Here's how the part is built. I have some questions about the finished solid (model axes, mm). A direction names the side the tool comes from. Coordinates: 2 decimals unless noted, no trailing zeros. Loops run counter-clockwise (first coordinate to the right, second up) from the corner with the lowest first, then second, coordinate; pieces in that order, holes last. Notation, with made-up numbers: M 24.5,51 L 47.5,51 A12 cw 47.5,58 Z; hole C -22,76.25 d1. An arc over 180 degrees is marked long. Use CSV: the item, a comma, the result in double quotes. Start each with the question number.
Q1. If we section it at A-A (z = -52): Please give me the cut outline in (x, y) (3 decimals), and give its area (3 significant figures).
Q2. For pin 1 Ø5 at (y, z) = (6, -34.5) entering from +X; pin 2 Ø1 at (x, y) = (971, 20) entering from -Z, each with a flat end and sliding along its axis, tell me the tip position at first contact or that it passes through.
Q3. If we mould it in two halves opening along Z, with no side actions, what happens to faces 1 (the flat face through (604, 22.225, -38)), 2 (the flat face through (37.9, 2.4, -38.3)), 3 (the flat face through (604, 25.4, -38))? For each: +Z half, -Z half, draft (parallel to the pull), parting line (faces both ways), or undercut.
Q4. If we section it at C-C (y = 12.25): Please give me the cut outline in (x, z) (3 decimals).
Q5. Please list where these lines run through material, in increasing order: probe 1 along Z at (x, y) = (878, 10) (3 decimals); probe 2 along Y at (x, z) = (584, -8) (3 decimals); probe 3 along Z at (x, y) = (941, 5.25). Write a range as [from, to].
Q6. If we section it at B-B (x = 89.5): Please give me the cut outline in (y, z) (3 decimals), and give its area (3 significant figures).
Q7. Which directions (+Z, -Z, +X, -X, +Y, -Y) give clear straight access to the entire face, cutting with the end or side of a thin tool? Please do faces 4 (the flat face through (604, 3.175, -38)), 5 (the flat face through (1219.2, 2, -38)).
from build123d import *

# Parameters (mm, degrees)
SKETCH1_W           = 76.2
SKETCH1_H           = 25.4
BOSS_EXTRUDE1_DEPTH = 1219.2
FILLET1_R           = 6.35
SHELL1_T            = -3.175
CUT_EXTRUDE1_DEPTH  = 25.4


with BuildPart() as part:
    # Sketch1 → Boss-Extrude1 (new body)
    with BuildSketch(Plane(origin=(0, 0, 0), x_dir=(0, 0, -1), z_dir=(1, 0, 0))):
        with Locations((38.1, 12.7)):
            Rectangle(SKETCH1_W, SKETCH1_H)
    extrude(amount=BOSS_EXTRUDE1_DEPTH)

    # Fillet1
    fillet1_edges = [part.edges().sort_by_distance(p)[0] for p in [
        (609.6, 25.4, 0),
        (609.6, 25.4, -76.2),
        (609.6, 0, -76.2),
        (609.6, 0, 0),
    ]]
    fillet(fillet1_edges, radius=FILLET1_R)

    # Shell1
    shell1_openings = [part.faces().sort_by_distance(p)[0] for p in [
        (1219.2, 12.7, -38.1),
        (0, 12.7, -38.1),
    ]]
    offset(amount=SHELL1_T, openings=shell1_openings, kind=Kind.INTERSECTION)

    # Sketch2 → Cut-Extrude1 (cut)
    with BuildSketch(Plane(origin=(0, 25.4, 0), x_dir=(1, 0, 0), z_dir=(0, 1, 0))):
        Polygon((0, 76.2), (76.2, 0), (0, 0), align=None)
    extrude(amount=-CUT_EXTRUDE1_DEPTH, mode=Mode.SUBTRACT)


solid = part.part
Results below:
1,outline,"M 24.2,0 L 1219.2,0 L 1219.2,3.175 L 24.2,3.175 Z; M 24.2,22.225 L 1219.2,22.225 L 1219.2,25.4 L 24.2,25.4 Z"
1,area,"7,590 mm^2"
2,pin 1,"through"
2,pin 2,"z = -76.18"
3,face 1,"undercut"
3,face 2,"+Z half"
3,face 3,"draft"
4,outline,"M 0,-76.2 L 1219.2,-76.2 L 1219.2,-73.025 L 3.175,-73.025 Z; M 73.025,-3.175 L 1219.2,-3.175 L 1219.2,0 L 76.2,0 Z"
5,probe 1,"[-76.2, -73.025], [-3.175, 0]"
5,probe 2,"[0, 3.175], [22.225, 25.4]"
5,probe 3,"[-76.1, -72.83], [-3.37, -0.1]"
6,outline,"M 0,-69.85 A6.35 ccw 6.35,-76.2 L 19.05,-76.2 A6.35 ccw 25.4,-69.85 L 25.4,-6.35 A6.35 ccw 19.05,0 L 6.35,0 A6.35 ccw 0,-6.35 Z; hole M 3.175,-69.85 A3.175 ccw 6.35,-73.025 L 19.05,-73.025 A3.175 ccw 22.225,-69.85 L 22.225,-6.35 A3.175 ccw 19.05,-3.175 L 6.35,-3.175 A3.175 ccw 3.175,-6.35 Z"
6,area,"579 mm^2"
7,face 4,"+X, -X"
7,face 5,"+Z, -Z, +X, +Y, -Y"
